```python
from build123d import *

# Parameters (mm, degrees)
BOSS_EXTRUDE1_DEPTH      = 7.5
BOSS_EXTRUDE1_DEPTH_BACK = 7.5
BOSS_EXTRUDE2_DEPTH      = 28.4
BOSS_EXTRUDE2_DEPTH_BACK = 22.4


with BuildPart() as part:
    # Sketch1 → Revolve1 (revolve)
    with BuildSketch(Plane(origin=(0, 0, 0), x_dir=(0, 0, -1), z_dir=(1, 0, 0))):
        Polygon((0, 0), (2, 0), (2, -22.5), (-80, -22.5), (-80, -20), (0, -20), align=None)
    revolve(axis=Axis((0, 0, 0), (0, 0, -1)))

    # Sketch3 → Boss-Extrude1 (add, two sides)
    with BuildSketch(Plane(origin=(0, 0, 48), x_dir=(-1, 0, 0), z_dir=(0, 0, -1))) as boss_extrude1_sk:
        with BuildLine():
            Line((-16.770509831, 15), (-22.770509831, 15))
            Line((-22.770509831, 15), (-22.770509831, -15))
            Line((-22.770509831, -15), (-16.770509831, -15))
            ThreePointArc((-16.770509831, -15), (-22.5, 0), (-16.770509831, 15))
        make_face()
    extrude(amount=BOSS_EXTRUDE1_DEPTH)
    extrude(boss_extrude1_sk.sketch, amount=-BOSS_EXTRUDE1_DEPTH_BACK)

    # Sketch4 → Boss-Extrude2 (add, two sides)
    with BuildSketch(Plane(origin=(0, 0, 48), x_dir=(-1, 0, 0), z_dir=(0, 0, -1))) as boss_extrude2_sk:
        with BuildLine():
            ThreePointArc((-20, 10.307764064), (0, 22.5), (20, 10.307764064))
            Line((20, 10.307764064), (20, 23.307764064))
            Line((20, 23.307764064), (-22.770509831, 23.307764064))
            Line((-22.770509831, 23.307764064), (-22.770509831, 15))
            Line((-22.770509831, 15), (-20, 15))
            Line((-20, 15), (-20, 10.307764064))
        make_face()
    extrude(amount=BOSS_EXTRUDE2_DEPTH)
    extrude(boss_extrude2_sk.sketch, amount=-BOSS_EXTRUDE2_DEPTH_BACK)


solid = part.part
```
Geometry: final body of the model. Coordinates: model frame, mm. A direction names the side the tool comes from. Coordinates: 2 decimals unless noted, no trailing zeros. Order: outer loops, then holes, each group sorted by start corner. A loop starts at its lowest first (then second) coordinate and runs counter-clockwise, first axis right, second up. Notation, with made-up numbers: (53, -24.5) - (105, -24.5) arc R6 cw to (105, -15.5) - close; hole circle Ø4 at (26, -2.75). An arc over 180 degrees is marked (long way). Write each question's results on one line, items separated by ' | '.
1) Section D-D, the plane z = 43.5. Return loops of the section in (x, y), plus the area to 3 significant figures.
Results list:
outline: (-20, 10.31) arc R22.5 ccw to (16.77, -15) - (22.77, -15) - (22.77, 23.31) - (-20, 23.31) - close; hole circle Ø40 at (0, 0) | area: 584 mm^2
2) Pin query (flat end, axial travel): pin 1 (5 mm diameter, centred on y = 13, z = 63.5, fed in from +X); pin 2 (4 mm diameter, centred on y = 12.5, z = 33.5, fed in from +X); pin 3 (3 mm diameter, centred on y = 12.5, z = 22, fed in from -X); pin 4 (6.5 mm diameter, centred on x = 21, z = 51.5, fed in from -Y). Return the tip coordinate at first contact, or that it passes through.
Results list:
pin 1: x = 22.77 | pin 2: x = 20 | pin 3: x = -20 | pin 4: y = -15
3) Section C-C, the plane y = 0. Return loops of the section in (x, z), plus the area to 3 significant figures.
Results list:
outline: (-22.5, -2) - (22.5, -2) - (22.5, 40.5) - (22.77, 40.5) - (22.77, 55.5) - (22.5, 55.5) - (22.5, 80) - (20, 80) - (20, 0) - (-20, 0) - (-20, 80) - (-22.5, 80) - close | area: 494 mm^2
4) Section B-B, the plane x = 0. Return loops of the section in (y, z).
Results list:
outline: (-22.5, -2) - (22.5, -2) - (22.5, 19.6) - (23.31, 19.6) - (23.31, 70.4) - (22.5, 70.4) - (22.5, 80) - (20, 80) - (20, 0) - (-20, 0) - (-20, 80) - (-22.5, 80) - close
5) Set-up query: faces 1 (the cylindrical face through (-6.76, -21.46, 39.57)), 2 (the flat face through (22.5, -3.3, 55.5)), 3 (the flat face through (20, 13, 30)), 4 (the cylindrical face through (19.524, 4.336, 39.44)), 5 (the flat face through (-20, 17, 45)). Return all of +Z, -Z, +X, -X, +Y, -Y with unobstructed straight access to the full face (end or side cutting, diameter ignored); none if empty.
Results list:
face 1: none | face 2: +Z, +X | face 3: -Z, +X | face 4: +Z | face 5: +Z, -Z, -X, +Y
6) Section A-A, the plane z = 20.5. Return loops of the section in (x, y), plus the area to 3 significant figures.
Results list:
outline: (-20, 10.31) arc R22.5 ccw (long way) to (20, 10.31) - (20, 15) - (22.77, 15) - (22.77, 23.31) - (-20, 23.31) - close; hole circle Ø40 at (0, 0) | area: 529 mm^2
7) Line query: line 1 (X direction, y = 0, z = 19); line 2 (Y direction, x = 0, z = 43); line 3 (Z direction, x = -7.5, y = 2). Output: solid intervals per line, ascending. Write a range as from..to.
Results list:
line 1: -22.5..-20, 20..22.5 | line 2: -22.5..-20, 20..23.31 | line 3: -2..0
8) Pull-direction query (Y, two-part tool) for faces 6 (the flat face through (1, 23.308, 45)), 7 (the flat face through (3, 23, 70.4)), 8 (the flat face through (20, 13, 63)); classes: pulls with the +Y half, pulls with the -Y half, needs draft (parallel to the pull), parting line crosses it, or undercut.
Results list:
face 6: pulls with the +Y half | face 7: needs draft | face 8: undercut
